Check sheet for the drawn part. Datum: minimum x, y, z corner. Units: mm. A direction names the side the tool comes from. Round coordinates to 2 decimals unless told otherwise and drop trailing zeros. Write each loop counter-clockwise with the first axis right and the second up, starting at its lowest first coordinate (ties: lowest second). Pieces come first, ordered by that corner, then holes. Notation, with made-up numbers: (-0.75, -22) - (37.25, -22) arc R18 cw to (37.25, 0) - close; hole circle Ø7 at (83.5, -15). An arc over 180 degrees is marked (long way). Answer as a JSON object with one key per item and string values. Group by question number.
Item 1: Sectioned sample at D-D on y = 13.5. Record the boundary of the cut face in (x, z).
Item 2: Gauge pin test, flat ends, axial feed: P1, Ø1, axis at x = 2, z = 26.5, coming from the +Y side; P2, Ø1.5, axis at x = 7.5, z = 18, coming from the +Y side; P3, Ø2.5, axis at x = 6, z = 18, coming from the -Y side; P4, Ø2.5, axis at y = 17.5, z = 6.5, coming from the +X side. Record the tip position at first contact, or that the pin passes through.
Item 3: Set-up check for the marked faces 1 and 2: record each of +Z, -Z, +X, -X, +Y, -Y from which the full face is reachable in a straight line by a thin tool's end or side.
Item 4: Sectioned sample at A-A on y = 17.5. Record the boundary of the cut face in (x, z).
Item 5: Sectioned sample at C-C on z = 28.5. Record the boundary of the cut face in (x, y).
Item 6: Thickness scan on line 1 (Y direction, x = 5, z = 17.5); line 2 (Y direction, x = 6, z = 28.5); line 3 (Z direction, x = 1, y = 17). Record the ranges inside material, lowest first.
Item 7: Sectioned sample at B-B on x = 4.75. Record the boundary of the cut face in (y, z), plus the area to 3 significant figures.
Item 8: Release check for a two-part mould opening along Z. For the marked faces 3, 4 and 5 record: pulls with the +Z half, pulls with the -Z half, needs draft (parallel to the pull), parting line crosses it, or undercut.
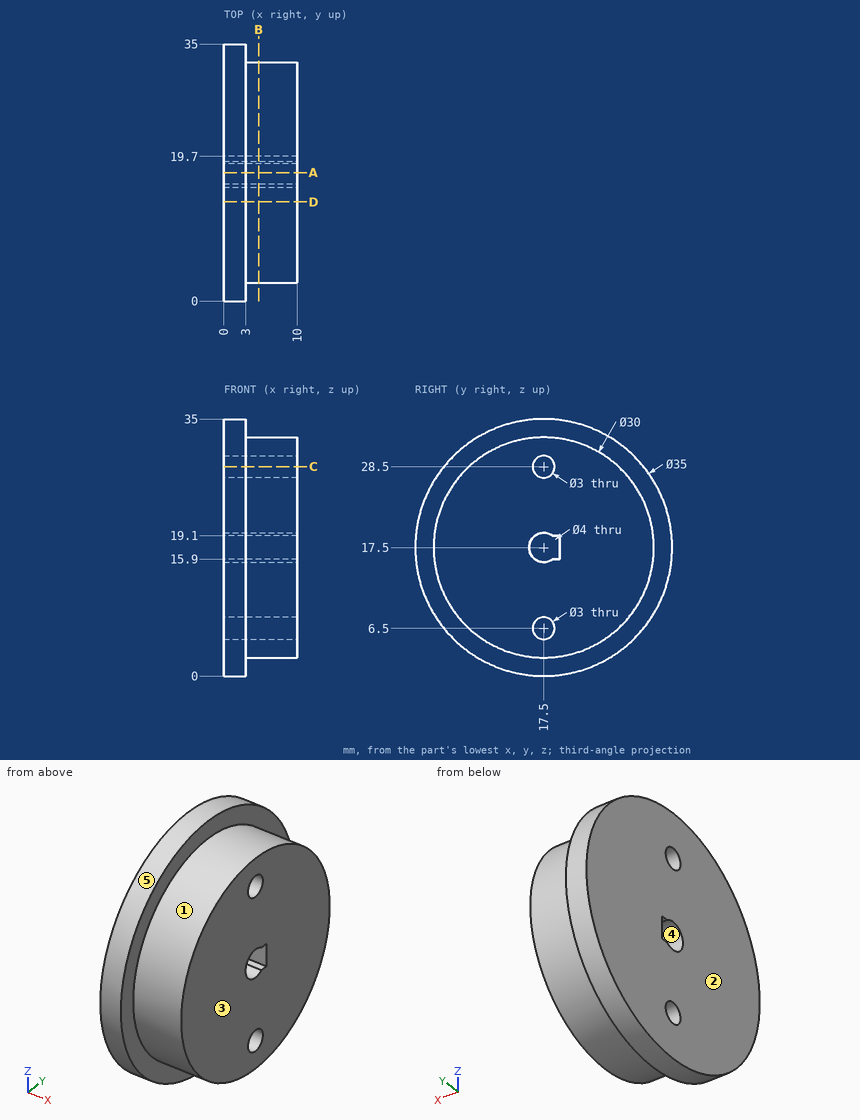
Completed:
{
 "1": {"outline": "(0, 0.46) - (3, 0.46) - (3, 3.04) - (10, 3.04) - (10, 31.96) - (3, 31.96) - (3, 34.54) - (0, 34.54) - close"},
 "2": {"P1": "y = 32.8", "P2": "y = 32.5", "P3": "y = 2.5", "P4": "through"},
 "3": {"face 1": "+X", "face 2": "+Z, -Z, -X, +Y, -Y"},
 "4": {"outline": "(0, 0) - (3, 0) - (3, 2.5) - (10, 2.5) - (10, 5) - (0, 5) - close; (0, 8) - (10, 8) - (10, 15.5) - (0, 15.5) - close; (0, 19.5) - (10, 19.5) - (10, 27) - (0, 27) - close; (0, 30) - (10, 30) - (10, 32.5) - (3, 32.5) - (3, 35) - (0, 35) - close"},
 "5": {"outline": "(0, 3.89) - (3, 3.89) - (3, 7.3) - (10, 7.3) - (10, 16) - (0, 16) - close; (0, 19) - (10, 19) - (10, 27.7) - (3, 27.7) - (3, 31.11) - (0, 31.11) - close"},
 "6": {"line 1": "2.5 to 15.5, 19.7 to 32.5", "line 2": "7.3 to 16, 19 to 27.7", "line 3": "0.01 to 5.09, 7.91 to 15.56, 19.44 to 27.09, 29.91 to 34.99"},
 "7": {"outline": "circle Ø30 at (17.5, 17.5); hole circle Ø3 at (17.5, 6.5); hole circle Ø3 at (17.5, 28.5); hole (18.7, 15.9) - (19.7, 15.9) - (19.7, 19.1) - (18.7, 19.1) arc R2 ccw (long way) to start", "area": "679 mm²"},
 "8": {"face 3": "needs draft", "face 4": "undercut", "face 5": "parting line crosses it"}
}
